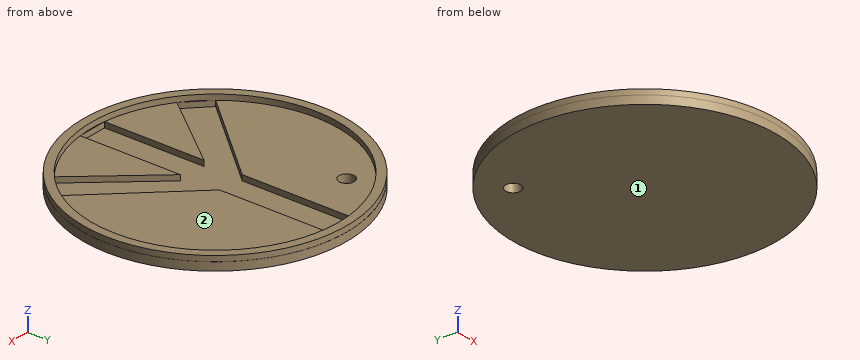
from build123d import *

# Parameters (mm, degrees)
F0_R     = 48.11598
F1_DEPTH = 3
F2_R     = 48.065002
F2_R_2   = 45.023817
F3_DEPTH = 2
F5_DEPTH = 2
F6_R     = 2.767495
F7_DEPTH = 3


with BuildPart() as f1:
    # F0 (on Top) → F1 (new body)
    with BuildSketch(Plane.XY):
        Circle(F0_R)
    extrude(amount=F1_DEPTH)

    # F2 (on face) → F3 (join)
    with BuildSketch(Plane.XY.offset(3)):
        Circle(F2_R)
        Circle(F2_R_2, mode=Mode.SUBTRACT)
    extrude(amount=F3_DEPTH)

    # F4 (on face) → F5 (cut)
    with BuildSketch(Plane.XY.offset(3)):
        Polygon((-6.218928, -8.945531), (-6.218928, -44.592253), (4.409318, -44.807388), (4.409318, -8.945531), (27.452203, -35.686421), (35.229265, -28.036458), (4.409318, 5.132682), (4.409318, 44.807388), (-6.452514, 44.559053), (-6.452514, 4.54609), (-35.229265, -28.036458), (-27.452203, -35.686421), align=None)
    extrude(amount=-F5_DEPTH, mode=Mode.SUBTRACT)

    # F6 (on face) → F7 (cut)
    with BuildSketch(Plane.XY.offset(3)):
        with Locations((-22.898344, 28.801464)):
            Circle(F6_R)
    extrude(amount=-F7_DEPTH, mode=Mode.SUBTRACT)


solid = f1.part
Here's how the part is built. I have some questions about the finished solid (model axes, mm). Face numbers are marked on the shaded views. Round coordinates to 2 decimals unless told otherwise and drop trailing zeros. Loops run counter-clockwise (first coordinate to the right, second up) from the corner with the lowest first, then second, coordinate; pieces in that order, holes last. Notation, with made-up numbers: (83, -13) -> (106, -13) arc R22 ccw to (106, 11) -> close; hole circle Ø10 at (-21.75, 26.5). An arc over 180 degrees is marked (long way). Write each question's results on one line, items separated by ' | '.
(1) If we section it at A-A, the plane x = -23: List the corners of the cut face in (y, z) for me.
Worked answers:
outline: (-42.26, 0) -> (26.04, 0) -> (26.04, 3) -> (-14.19, 3) -> (-14.19, 1) -> (-30.08, 1) -> (-30.08, 3) -> (-38.71, 3) -> (-38.71, 5) -> (-42.2, 5) -> (-42.2, 3) -> (-42.26, 3) -> close; (31.57, 0) -> (42.26, 0) -> (42.26, 3) -> (42.2, 3) -> (42.2, 5) -> (38.71, 5) -> (38.71, 3) -> (31.57, 3) -> close
(2) If I drill on L1, parallel to Y at x = 0, z = 4.2 (3 decimals); L2, parallel to Y at x = -21.5, z = 2.2; L3, parallel to X at y = -12, z = 2.8, over which ranges is the centre line in solid material (lowest first)?
Worked answers:
L1: -48.065 to -45.024, 45.024 to 48.065 | L2: -43.05 to -28.19, -12.49 to 26.41, 31.19 to 43.05 | L3: -46.6 to -21.07, -8.64 to -6.22, 4.41 to 7.04, 20.33 to 46.6
(3) We'd pull the mould along Y, two halves only. Please class the marked faces 1 and 2: released by +Y, released by -Y, zero draft, split by the parting line, or undercut.
Worked answers:
face 1: zero draft | face 2: undercut
(4) If we section it at D-D, the plane x = 0: List the corners of the cut face in (y, z) for me (3 decimals), then the cut area to 3 significant figures.
Worked answers:
outline: (-48.116, 0) -> (48.116, 0) -> (48.116, 3) -> (48.065, 3) -> (48.065, 5) -> (45.024, 5) -> (45.024, 3) -> (44.707, 3) -> (44.707, 1) -> (-44.718, 1) -> (-44.718, 3) -> (-45.024, 3) -> (-45.024, 5) -> (-48.065, 5) -> (-48.065, 3) -> (-48.116, 3) -> close | area: 122 mm2
(5) If we section it at B-B, the plane y = 0: List the corners of the cut face in (x, z) for me (3 decimals), then the cut area to 3 significant figures.
Worked answers:
outline: (-48.116, 0) -> (48.116, 0) -> (48.116, 3) -> (48.065, 3) -> (48.065, 5) -> (45.024, 5) -> (45.024, 3) -> (9.178, 3) -> (9.178, 1) -> (-10.468, 1) -> (-10.468, 3) -> (-45.024, 3) -> (-45.024, 5) -> (-48.065, 5) -> (-48.065, 3) -> (-48.116, 3) -> close | area: 262 mm2
(6) For P1, Ø2, axis at y = 19.5, z = 2, coming from the +X side; P2, Ø19.5, axis at x = -24.5, y = 8.5, coming from the +Z side; P3, Ø2, axis at y = 28, z = 1.5, coming from the -X side; P4, Ø4.5, axis at x = -22.9, y = 28.8, coming from the +Z side, each with a flat end and sliding along its axis, tell me the tip position at first contact or that it passes through.
Worked answers:
P1: x = 44.42 | P2: z = 3 | P3: x = -39.83 | P4: through
(7) If we section it at C-C, the plane z = 3.85: List the corners of the cut face in (x, y) for me (3 decimals).
Worked answers:
outline: circle Ø96.13 at (0, 0); hole circle Ø90.048 at (0, 0)
